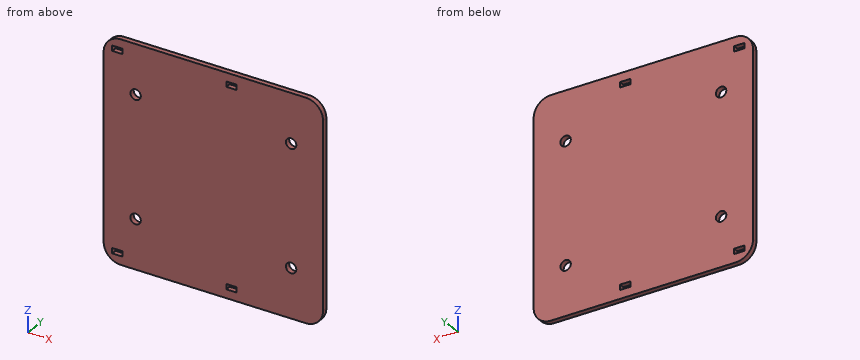
```python
from build123d import *

# Parameters (mm, degrees)
SKETCH1_R           = 3
BOSS_EXTRUDE1_DEPTH = 3
CUT_EXTRUDE1_REACH  = 91.853
SKETCH2_W           = 6.05
SKETCH2_H           = 3.05
FILLET1_R           = 0.1


with BuildPart() as part:
    # Sketch1 → Boss-Extrude1 (new body)
    with BuildSketch(Plane(origin=(0, 0, 0), x_dir=(1, 0, 0), z_dir=(0, 1, 0))):
        with BuildLine():
            Line((-53.5, 63.5), (53.5, 63.5))
            ThreePointArc((53.5, 63.5), (60.571067812, 60.571067812), (63.5, 53.5))
            Line((63.5, 53.5), (63.5, -53.5))
            ThreePointArc((63.5, -53.5), (60.571067812, -60.571067812), (53.5, -63.5))
            Line((53.5, -63.5), (-53.5, -63.5))
            ThreePointArc((-53.5, -63.5), (-60.571067812, -60.571067812), (-63.5, -53.5))
            Line((-63.5, -53.5), (-63.5, 53.5))
            ThreePointArc((-63.5, 53.5), (-60.571067812, 60.571067812), (-53.5, 63.5))
        make_face()
        with Locations(Location((-45, 35, 0), (0, 0, 270))):
            Circle(SKETCH1_R, mode=Mode.SUBTRACT)
        with Locations(Location((45, 35, 0), (0, 0, 90))):
            Circle(SKETCH1_R, mode=Mode.SUBTRACT)
        with Locations(Location((45, -35, 0), (0, 0, 270))):
            Circle(SKETCH1_R, mode=Mode.SUBTRACT)
        with Locations(Location((-45, -35, 0), (0, 0, 90))):
            Circle(SKETCH1_R, mode=Mode.SUBTRACT)
    extrude(amount=BOSS_EXTRUDE1_DEPTH)

    # Sketch2 → Cut-Extrude1 (cut, up to next)
    with BuildSketch(Plane(origin=(0, 3, 0), x_dir=(1, 0, 0), z_dir=(0, 1, 0)), mode=Mode.PRIVATE) as cut_extrude1_sk1:
        with Locations((-55.5, -57)):
            Rectangle(SKETCH2_W, SKETCH2_H)
    cut_extrude1_tool1 = extrude(cut_extrude1_sk1.sketch, amount=-CUT_EXTRUDE1_REACH, mode=Mode.PRIVATE) & part.part
    # Sketch2 → Cut-Extrude1 (cut, up to next)
    with BuildSketch(Plane(origin=(0, 3, 0), x_dir=(1, 0, 0), z_dir=(0, 1, 0)), mode=Mode.PRIVATE) as cut_extrude1_sk2:
        with Locations((10.5, -57)):
            Rectangle(SKETCH2_W, SKETCH2_H)
    cut_extrude1_tool2 = extrude(cut_extrude1_sk2.sketch, amount=-CUT_EXTRUDE1_REACH, mode=Mode.PRIVATE) & part.part
    # Sketch2 → Cut-Extrude1 (cut, up to next)
    with BuildSketch(Plane(origin=(0, 3, 0), x_dir=(1, 0, 0), z_dir=(0, 1, 0)), mode=Mode.PRIVATE) as cut_extrude1_sk3:
        with Locations((10.5, 57)):
            Rectangle(SKETCH2_W, SKETCH2_H)
    cut_extrude1_tool3 = extrude(cut_extrude1_sk3.sketch, amount=-CUT_EXTRUDE1_REACH, mode=Mode.PRIVATE) & part.part
    # Sketch2 → Cut-Extrude1 (cut, up to next)
    with BuildSketch(Plane(origin=(0, 3, 0), x_dir=(1, 0, 0), z_dir=(0, 1, 0)), mode=Mode.PRIVATE) as cut_extrude1_sk4:
        with Locations((-55.5, 57)):
            Rectangle(SKETCH2_W, SKETCH2_H)
    cut_extrude1_tool4 = extrude(cut_extrude1_sk4.sketch, amount=-CUT_EXTRUDE1_REACH, mode=Mode.PRIVATE) & part.part
    add(cut_extrude1_tool1.solids().sort_by_distance((-55.5, 3, 57))[0], mode=Mode.SUBTRACT)
    add(cut_extrude1_tool2.solids().sort_by_distance((10.5, 3, 57))[0], mode=Mode.SUBTRACT)
    add(cut_extrude1_tool3.solids().sort_by_distance((10.5, 3, -57))[0], mode=Mode.SUBTRACT)
    add(cut_extrude1_tool4.solids().sort_by_distance((-55.5, 3, -57))[0], mode=Mode.SUBTRACT)

    # Fillet1
    fillet1_edges = [part.edges().sort_by_distance(p)[0] for p in [
        (13.525, 1.5, -58.525),
        (13.525, 1.5, -55.475),
        (7.475, 1.5, -55.475),
        (7.475, 1.5, -58.525),
        (-58.525, 1.5, 58.525),
        (-58.525, 1.5, 55.475),
        (-52.475, 1.5, 55.475),
        (-52.475, 1.5, 58.525),
        (13.525, 1.5, 55.475),
        (13.525, 1.5, 58.525),
        (7.475, 1.5, 58.525),
        (7.475, 1.5, 55.475),
        (-58.525, 1.5, -55.475),
        (-58.525, 1.5, -58.525),
        (-52.475, 1.5, -58.525),
        (-52.475, 1.5, -55.475),
    ]]
    fillet(fillet1_edges, radius=FILLET1_R)


solid = part.part
```
Input: part model. Units: mm. Frame: model coordinates. Round coordinates to 2 decimals unless told otherwise and drop trailing zeros. Order: outer loops, then holes, each group sorted by start corner. A loop starts at its lowest first (then second) coordinate and runs counter-clockwise, first axis right, second up. Notation, with made-up numbers: (-31, 49) - (13, 49) arc R4 cw to (13, 54) - close; hole circle Ø11 at (-11.75, -22). An arc over 180 degrees is marked (long way). One line per question, with ' | ' between items. Start each with the question number.
1) Cut plane B-B, the plane x = -45. Return the cut outline in (y, z), then the cut area to 3 significant figures.
2) Contact query for flat-ended pins moving along their axis: P1, Ø0.9, axis at y = 2, z = -57.5, coming from the -X side; P2, Ø0.9, axis at x = -57, y = 1, coming from the +Z side. Output: stop coordinate, or through.
3) Ray query, probe 1 along X at (y, z) = (1.65, -35); probe 2 along X at (y, z) = (1.1, 36); probe 3 along Z at (x, y) = (-57, 1.4) (1 decimal). Return the intervals inside material, ascending.
4) Cut plane A-A, the plane z = 35. Return the cut outline in (x, y).
5) Cut plane C-C, the plane y = 1.2. Give the number of separate pieces and of enclosed holes in the cut face, then the cut area to 3 significant figures.
Worked out:
1) outline: (0, -63.5) - (3, -63.5) - (3, -38) - (0, -38) - close; (0, -32) - (3, -32) - (3, 32) - (0, 32) - close; (0, 38) - (3, 38) - (3, 63.5) - (0, 63.5) - close | area: 345 mm^2
2) P1: stops at x = -62.85 | P2: stops at z = 63.02
3) probe 1: x = -63.5 to -48, -42 to 42, 48 to 63.5 | probe 2: x = -63.5 to -47.83, -42.17 to 42.17, 47.83 to 63.5 | probe 3: z = -62.9 to -58.5, -55.5 to 55.5, 58.5 to 62.9
4) outline: (-63.5, 0) - (-48, 0) - (-48, 3) - (-63.5, 3) - close; (-42, 0) - (42, 0) - (42, 3) - (-42, 3) - close; (48, 0) - (63.5, 0) - (63.5, 3) - (48, 3) - close
5) separate pieces: 1 | enclosed holes: 8 | area: 15,900 mm^2
